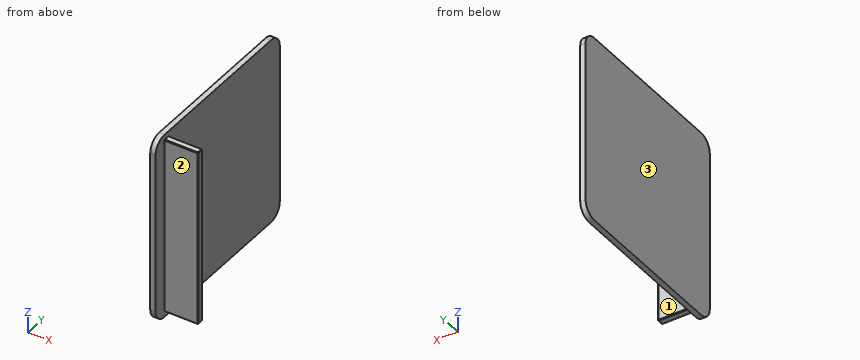
```python
from build123d import *

# Parameters (mm, degrees)
SKETCH_1_W      = 140
SKETCH_1_H      = 140
EXTRUDE_1_DEPTH = 4
SKETCH_3_W      = 132
SKETCH_3_H      = 5
EXTRUDE_2_DEPTH = 25
CHAMFER_1_SIZE  = 0.5
CHAMFER_2_SIZE  = 0.5
FILLET_1_R      = 10


with BuildPart() as part:
    # 草图1 → 凸台-拉伸1 (new body)
    with BuildSketch(Plane(origin=(0, 0, 0), x_dir=(0, 0, -1), z_dir=(1, 0, 0))):
        Rectangle(SKETCH_1_W, SKETCH_1_H)
    extrude(amount=EXTRUDE_1_DEPTH)

    # 草图3 → 凸台-拉伸2 (add)
    with BuildSketch(Plane(origin=(4, 0, 0), x_dir=(0, 0, -1), z_dir=(1, 0, 0))):
        with Locations((0, -57.5)):
            Rectangle(SKETCH_3_W, SKETCH_3_H)
    extrude(amount=EXTRUDE_2_DEPTH)

    # 倒角1
    chamfer_1_edges = [part.edges().sort_by_distance(p)[0] for p in [
        (29, -57.5, 66),
        (29, -60, 0),
        (29, -57.5, -66),
        (29, -55, 0),
    ]]
    chamfer(chamfer_1_edges, length=CHAMFER_1_SIZE)

    # 倒角2
    chamfer_2_edges = [part.edges().sort_by_distance(p)[0] for p in [
        (16.25, -55, 66),
        (16.25, -55, -66),
        (16.25, -60, -66),
        (16.25, -60, 66),
    ]]
    chamfer(chamfer_2_edges, length=CHAMFER_2_SIZE)

    # 圆角1
    fillet_1_edges = [part.edges().sort_by_distance(p)[0] for p in [
        (2, 70, 70),
        (2, 70, -70),
        (2, -70, -70),
        (2, -70, 70),
    ]]
    fillet(fillet_1_edges, radius=FILLET_1_R)


solid = part.part
```
Work out the finished part from the listing and answer in its coordinate system (mm). Face numbers are marked on the shaded views. A direction names the side the tool comes from. Coordinates: 2 decimals unless noted, no trailing zeros. Write each loop counter-clockwise with the first axis right and the second up, starting at its lowest first coordinate (ties: lowest second). Pieces come first, ordered by that corner, then holes.
Q1. A cutting plane is placed at C-C, the plane y = -49.5. Give the vertices of the cut face in (x, z).
Q2. Which of the six approach directions +Z, -Z, +X, -X, +Y, -Y give full straight-line access (tool end or side, diameter ignored) to the marked faces 1, 2 and 3?
Q3. A cutting plane is placed at B-B, the plane x = 21. Give the vertices of the cut face in (y, z), then the cut area to 4 significant figures.
Q4. Find the intervals of material crossed by line 1 (X direction, y = 45, z = 32); line 2 (Y direction, x = 16, z = -44.5), in increasing order.
Q5. Each of these flat-tipped pins is pushed along its axis until it touches: pin 1 Ø1 at (y, z) = (16.5, 40) entering from +X; pin 2 Ø3 at (x, y) = (20, -58.5) entering from +Z; pin 3 Ø1.2 at (x, y) = (11, -58) entering from -Z; pin 4 Ø4 at (y, z) = (-8, 24.5) entering from -X. Where does it stop, or does it pass through?
Q6. A cutting plane is placed at A-A, the plane z = -35. Give the vertices of the cut face in (x, y), then the cut area to 3 significant figures.
Findings below:
1. outline: (0, -70) - (4, -70) - (4, 70) - (0, 70) - close
2. face 1: +Z, -Z, +X, +Y
2. face 2: +Z, -Z, +X, -Y
2. face 3: +Z, -Z, -X, +Y, -Y
3. outline: (-60, -65.5) - (-59.5, -66) - (-55.5, -66) - (-55, -65.5) - (-55, 65.5) - (-55.5, 66) - (-59.5, 66) - (-60, 65.5) - close
3. area: 659.5 mm2
4. line 1: x = 0 to 4
4. line 2: y = -60 to -55
5. pin 1: stops at x = 4
5. pin 2: stops at z = 66
5. pin 3: stops at z = -66
5. pin 4: stops at x = 0
6. outline: (0, -70) - (4, -70) - (4, -60) - (28.5, -60) - (29, -59.5) - (29, -55.5) - (28.5, -55) - (4, -55) - (4, 70) - (0, 70) - close
6. area: 685 mm2
